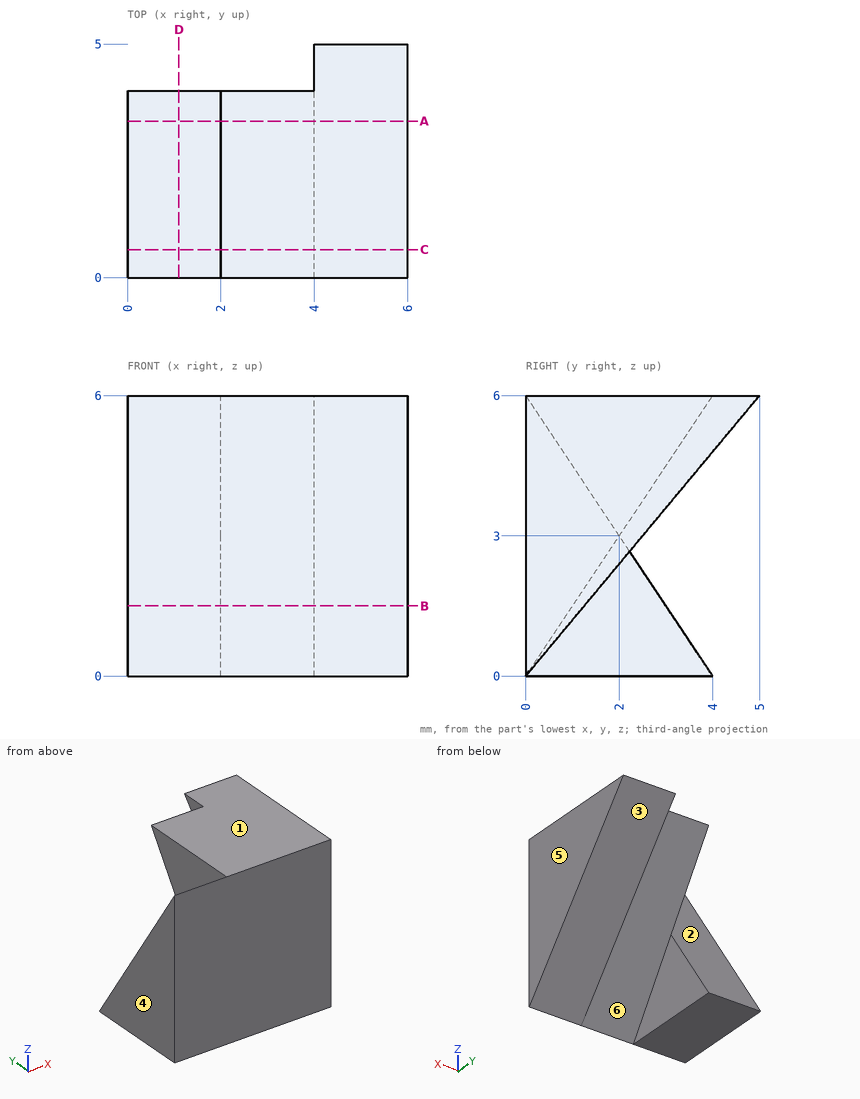
Answer from the drawing. Dimensions are ordinates in mm from the lowest x, y and z of the part. A direction names the side the tool comes from. Coordinates: 2 decimals unless noted, no trailing zeros. Write each loop counter-clockwise with the first axis right and the second up, starting at its lowest first coordinate (ties: lowest second). Pieces come first, ordered by that corner, then holes. Notation, with made-up numbers: M -20.75,50.5 L 26.25,50.5 A25 ccw 26.25,68.5 Z; hole C 27.5,47 d3. An arc over 180 degrees is marked long. Use a Markdown table: item, result.
Q1. Straight lines are drawn through the part: L1, parallel to X at y = 1.45, z = 1.8; L2, parallel to X at y = 0.95, z = 5.7; L3, parallel to Y at x = 2.3, z = 2.9. For each, find the intervals that lie inside material, in ascending order. Write a range as [from, to].
Answer block:
| item | result |
|---|---|
| L1 | x = [0, 2], [4, 6] |
| L2 | x = [2, 6] |
| L3 | y = [0, 1.93] |
Q2. The part is cut by section B-B, the plane z = 1.5. Write down the section's boundary in (x, y).
Answer block:
| item | result |
|---|---|
| outline | M 0,0 L 6,0 L 6,1.25 L 4,1.25 L 4,1 L 2,1 L 2,3 L 0,3 Z |
Q3. The part is cut by section A-A, the plane y = 3.35. Write down the section's boundary in (x, z) (3 decimals), then the cut area to 3 significant figures.
Answer block:
| item | result |
|---|---|
| outline | M 0,0 L 2,0 L 2,0.975 L 0,0.975 Z; M 2,5.025 L 4,5.025 L 4,4.02 L 6,4.02 L 6,6 L 2,6 Z |
| area | 7.86 mm2 |
Q4. Determine the mould class of the marked faces 3, 4, 5 and 6 for opening direction X: released by +X, released by -X, zero draft, split by the parting line, or undercut.
Answer block:
| item | result |
|---|---|
| face 3 | zero draft |
| face 4 | released by -X |
| face 5 | released by +X |
| face 6 | undercut |
Q5. The part is cut by section C-C, the plane y = 0.6. Write down the section's boundary in (x, z), then the cut area to 3 significant figures.
Answer block:
| item | result |
|---|---|
| outline | M 0,0 L 2,0 L 2,0.9 L 4,0.9 L 4,0.72 L 6,0.72 L 6,6 L 2,6 L 2,5.1 L 0,5.1 Z |
| area | 31.0 mm2 |
Q6. The part is cut by section D-D, the plane x = 1.1. Write down the section's boundary in (y, z), then the cut area to 3 significant figures.
Answer block:
| item | result |
|---|---|
| outline | M 0,0 L 4,0 L 0,6 Z |
| area | 12.0 mm2 |
Q7. Which of the six approach directions +Z, -Z, +X, -X, +Y, -Y give full straight-line access (tool end or side, diameter ignored) to the marked faces 1 and 2?
Answer block:
| item | result |
|---|---|
| face 1 | +Z, +X, -X, +Y, -Y |
| face 2 | +Z, -X, +Y |
